Work out the finished part from the listing and answer in its coordinate system (mm). Face numbers are marked on the shaded views. A direction names the side the tool comes from. Coordinates: 2 decimals unless noted, no trailing zeros. Order: outer loops, then holes, each group sorted by start corner. A loop starts at its lowest first (then second) coordinate and runs counter-clockwise, first axis right, second up. Notation, with made-up numbers: M -28.5,71.5 L -18.5,71.5 A8 cw -18.5,82.5 Z; hole C 83.25,-14 d10. An arc over 180 degrees is marked long. Use a Markdown table: item, result.
from build123d import *

# Parameters (mm, degrees)
SKETCH_W        = 21
SKETCH_H        = 19.7
PAD_DEPTH       = 75.9
FILLET_R        = 5
SKETCH001_W     = 21
SKETCH001_H     = 72.3
POCKET_DEPTH    = 8.6
SKETCH002_W     = 18.2
SKETCH002_H     = 72.3
POCKET001_DEPTH = 9.6
SKETCH003_R     = 1.6
POCKET002_DEPTH = 5
CHAMFER_SIZE    = 1


with BuildPart() as part:
    # Sketch → Pad (new body)
    with BuildSketch(Plane.XY):
        with Locations((0, 9.85)):
            Rectangle(SKETCH_W, SKETCH_H)
    extrude(amount=PAD_DEPTH)

    # Fillet
    fillet_edges = [part.edges().sort_by_distance(p)[0] for p in [
        (-10.5, 19.7, 37.95),
        (10.5, 19.7, 37.95),
    ]]
    fillet(fillet_edges, radius=FILLET_R)

    # Sketch001 (on Face6 of Fillet) → Pocket (cut)
    with BuildSketch(Plane(origin=(0, 19.7, 0), x_dir=(-1, 0, 0), z_dir=(0, 1, 0))):
        with Locations((0, 37.95)):
            Rectangle(SKETCH001_W, SKETCH001_H)
    extrude(amount=-POCKET_DEPTH, mode=Mode.SUBTRACT)

    # Sketch002 (on Face4 of Pocket) → Pocket001 (cut)
    with BuildSketch(Plane(origin=(0, 11.1, 0), x_dir=(-1, 0, 0), z_dir=(0, 1, 0))):
        with Locations((0, 37.95)):
            Rectangle(SKETCH002_W, SKETCH002_H)
    extrude(amount=-POCKET001_DEPTH, mode=Mode.SUBTRACT)

    # Sketch003 (on Face20 of Pocket001) → Pocket002 (cut)
    with BuildSketch(Plane(origin=(0, 1.5, 0), x_dir=(-1, 0, 0), z_dir=(0, 1, 0))):
        with Locations((0, 37.95)):
            Circle(SKETCH003_R)
    extrude(amount=-POCKET002_DEPTH, mode=Mode.SUBTRACT)

    # Chamfer
    chamfer_edges = [part.edges().sort_by_distance(p)[0] for p in [
        (1.6, 1.5, 37.95),
    ]]
    chamfer(chamfer_edges, length=CHAMFER_SIZE)


solid = part.part
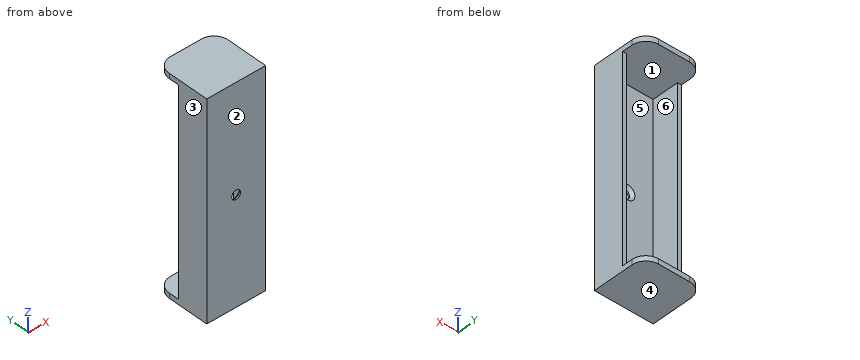
1. Find the intervals of material crossed by probe 1 along Z at (x, y) = (-3.25, 5); probe 2 along X at (y, z) = (1.75, 71.5); probe 3 along Z at (x, y) = (0, 0.1), in increasing order.
Answers below:
| item | result |
|---|---|
| probe 1 | 0 to 1.8, 74.1 to 75.9 |
| probe 2 | -10.5 to -9.1, 9.1 to 10.5 |
| probe 3 | 0 to 36.35, 39.55 to 75.9 |
2. For a pull along Z with two mould halves and no side action, classify the marked faces 3, 4, 5 and 6 as +Z half, -Z half, draft (parallel to the pull), parting line (faces both ways), or undercut.
Answers below:
| item | result |
|---|---|
| face 3 | draft |
| face 4 | -Z half |
| face 5 | undercut |
| face 6 | undercut |
3. Section C-C on z = 37.95 is taken. Determine the outline of the cut face in (x, y).
Answers below:
| item | result |
|---|---|
| outline | M -10.5,0 L -1.6,0 L -1.6,0.5 L -2.6,1.5 L -9.1,1.5 L -9.1,11.1 L -10.5,11.1 Z; M 1.6,0 L 10.5,0 L 10.5,11.1 L 9.1,11.1 L 9.1,1.5 L 2.6,1.5 L 1.6,0.5 Z |
4. Section A-A on y = 13 is taken. Determine the outline of the cut face in (x, z), then the cut area to 3 significant figures.
Answers below:
| item | result |
|---|---|
| outline | M -10.5,0 L 10.5,0 L 10.5,1.8 L -10.5,1.8 Z; M -10.5,74.1 L 10.5,74.1 L 10.5,75.9 L -10.5,75.9 Z |
| area | 75.6 mm² |
5. For the marked faces 1 and 2, determine the directions among +Z, -Z, +X, -X, +Y, -Y from which every point of the face is accessible in a straight line to the end or side of a thin tool.
Answers below:
| item | result |
|---|---|
| face 1 | +Y |
| face 2 | +Z, -Z, +X, -X, -Y |
6. Flat-ended cylindrical pins translate along their axes: P1, Ø0.7, axis at x = -10, z = 30.5, coming from the +Y side; P2, Ø1, axis at x = 5, z = 45, coming from the +Y side; P3, Ø3, axis at x = 0, z = 37.95, coming from the -Y side (3 decimals). Find the tip coordinate at first contact, or state that the pin passes through.
Answers below:
| item | result |
|---|---|
| P1 | y = 11.1 |
| P2 | y = 1.5 |
| P3 | through |
7. Section D-D on z = 46 is taken. Determine the outline of the cut face in (x, y).
Answers below:
| item | result |
|---|---|
| outline | M -10.5,0 L 10.5,0 L 10.5,11.1 L 9.1,11.1 L 9.1,1.5 L -9.1,1.5 L -9.1,11.1 L -10.5,11.1 Z |
8. Section B-B on x = 0 is taken. Determine the outline of the cut face in (y, z).
Answers below:
| item | result |
|---|---|
| outline | M 0,0 L 19.7,0 L 19.7,1.8 L 1.5,1.8 L 1.5,35.35 L 0.5,36.35 L 0,36.35 Z; M 0,39.55 L 0.5,39.55 L 1.5,40.55 L 1.5,74.1 L 19.7,74.1 L 19.7,75.9 L 0,75.9 Z |
